from build123d import *

# Parameters (mm, degrees)
F0_R     = 3.25
F1_DEPTH = 10
F3_DEPTH = 1


with BuildPart() as f1:
    # F0 (on Top) → F1 (new body)
    with BuildSketch(Plane.XY):
        Circle(F0_R)
    extrude(amount=F1_DEPTH)

    # F2 (on face) → F3 (cut)
    with BuildSketch(Plane.XY.offset(10)):
        with BuildLine():
            Line((6.379369, 0), (3.25, 0))
            ThreePointArc((3.25, 0), (2.298097, -2.298097), (0, -3.25))
            Line((0, -3.25), (0, -5.629462))
            Line((0, -5.629462), (6.379369, -5.629462))
            Line((6.379369, -5.629462), (6.379369, 0))
        make_face()
        with BuildLine():
            Line((3.25, 0), (0, 0))
            Line((0, 0), (0, -3.25))
            ThreePointArc((0, -3.25), (2.298097, -2.298097), (3.25, 0))
        make_face()
    extrude(amount=-F3_DEPTH, mode=Mode.SUBTRACT)


with BuildPart() as f4_1:
    # F4: copy of F1
    add(f1.part)


with BuildPart() as f5_1:
    # F5: copy of F4_1
    add(f4_1.part)


with BuildPart() as f6_1:
    # F6: copy of F5_1
    add(f5_1.part)


with BuildPart() as f7_1:
    # F7: copy of F6_1
    add(f6_1.part)


with BuildPart() as f8_1:
    # F8: copy of F7_1
    add(f7_1.part)


with BuildPart() as f9_1:
    # F9: copy of F8_1
    add(f8_1.part)


with BuildPart() as f10_1:
    # F10: copy of F9_1
    add(f9_1.part)


with BuildPart() as f11_1:
    # F11: copy of F1
    add(f1.part)


solid = f1.part
Input: part model. Units: mm. Frame: model coordinates. A direction names the side the tool comes from. Round coordinates to 2 decimals unless told otherwise and drop trailing zeros. Write each loop counter-clockwise with the first axis right and the second up, starting at its lowest first coordinate (ties: lowest second). Pieces come first, ordered by that corner, then holes.
1) Cut plane D-D (x = -2). Return the cut outline in (y, z).
2) Cut plane B-B (y = -0.25). Return the cut outline in (x, z), then the cut area to 3 significant figures.
3) Reachability of faces 1 (the flat face through (0, -1.6, 9.5)), 2 (the cylindrical face through (-2.395, 2.197, 4.93)) from +Z, -Z, +X, -X, +Y, -Y: full face, straight path, thin tool, end or side. Return the list, or none.
4) Contact query for flat-ended pins moving along their axis: P1, Ø2.5, axis at x = 1.5, y = -1.5, coming from the +Z side; P2, Ø0.5, axis at x = 1, z = 9.5, coming from the -Y side; P3, Ø0.5, axis at y = -2.5, z = 9.5, coming from the +X side. Output: stop coordinate, or through.
5) Cut plane A-A (z = 0.75). Return the cut outline in (x, y).
6) Cut plane C-C (x = 0.75). Return the cut outline in (y, z), then the cut area to 3 significant figures.
7) Ray query, L1, parallel to Z at x = 0.75, y = -1; L2, parallel to X at y = 0.25, z = 5; L3, parallel to Y at x = -1.5, z = 7. Return the intervals inside material, ascending.
Geometry says:
1. outline: (-2.56, 0) - (2.56, 0) - (2.56, 10) - (-2.56, 10) - close
2. outline: (-3.24, 0) - (3.24, 0) - (3.24, 9) - (0, 9) - (0, 10) - (-3.24, 10) - close
2. area: 61.6 mm2
3. face 1: +Z, +X, -Y
3. face 2: +Z, -Z
4. P1: stops at z = 9
4. P2: stops at y = 0
4. P3: stops at x = 0
5. outline: circle Ø6.5 at (0, 0)
6. outline: (-3.16, 0) - (3.16, 0) - (3.16, 10) - (0, 10) - (0, 9) - (-3.16, 9) - close
6. area: 60.1 mm2
7. L1: z = 0 to 9
7. L2: x = -3.24 to 3.24
7. L3: y = -2.88 to 2.88
